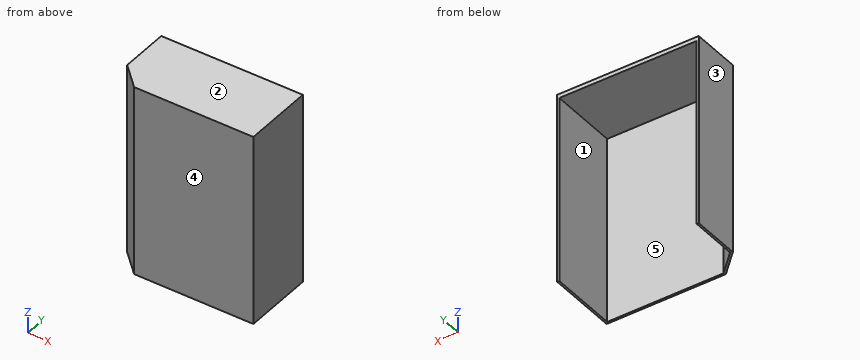
from build123d import *

# Parameters (mm, degrees)
F1_DEPTH = 900
F3_DEPTH = 20


with BuildPart() as f1:
    # F0 (on Top) → F1 (new body)
    with BuildSketch(Plane.XY):
        Polygon((0, 100), (0, 330), (-10, 330), (-10, 95.789346), (95.926052, -7.69314), (670, -7.69314), (670, 332.30686), (660, 332.30686), (660, 2.30686), (100, 2.30686), align=None)
    extrude(amount=F1_DEPTH)

    # F2 (on face) → F3 (join)
    with BuildSketch(Plane.XY.offset(900)):
        Polygon((670, 332.30686), (-10, 330), (-10, 95.789346), (95.926052, -7.69314), (670, -7.69314), align=None)
    extrude(amount=F3_DEPTH)


solid = f1.part
Here's how the part is built. I have some questions about the finished solid (model axes, mm). Face numbers are marked on the shaded views. A direction names the side the tool comes from. Give positions to 0.01 mm unless a question says otherwise; leave off trailing zeros. Order: outer loops, then holes, each group sorted by start corner. A loop starts at its lowest first (then second) coordinate and runs counter-clockwise, first axis right, second up. Notation, with made-up numbers: (-4.75, 6) -> (6.25, 6) arc R26 cw to (6.25, 26) -> close; hole circle Ø10 at (29.5, 12). An arc over 180 degrees is marked (long way). Use a Markdown table: item, result. Add a question column.
Item 1: Imagine slicing it at A-A on y = 229. Please give me the cut outline in (x, z), plus the area to 3 significant figures.
Item 2: Will these pins go through, and if not, where does the flat tip stop? pin 1 (3 mm diameter, centred on x = 111.5, y = 177.5, fed in from -Z); pin 2 (5 mm diameter, centred on x = 320.5, z = 785, fed in from +Y); pin 3 (5 mm diameter, centred on x = -5.5, z = 568.5, fed in from +Y).
Item 3: If we mould it in two halves opening along X, with no side actions, what happens to the marked faces 1, 2 and 3? For each: pulls with the +X half, pulls with the -X half, needs draft (parallel to the pull), parting line crosses it, or undercut.
Item 4: Imagine slicing it at B-B on z = 842. Please give me the cut outline in (x, y), plus the area to 3 significant figures.
Item 5: I need wall thicknesses on line 1 (X direction, y = 127, z = 623.5); line 2 (Y direction, x = 106, z = 616.5); line 3 (Z direction, x = 476.5, y = 151). Which ranges of each line are inside material? Lowest first, please.
Item 6: Imagine slicing it at D-D on x = 461. Please give me the cut outline in (y, z), plus the area to 3 significant figures.
Item 7: Imagine slicing it at C-C on x = 320.5. Please give me the cut outline in (y, z), plus the area to 3 significant figures.
Item 8: For the marked faces 4 and 5, which set-ups out of +Z, -Z, +X, -X, +Y, -Y let a thin tool reach every point of the face, with its end or its side?
Data:
| question | item | result |
|---|---|---|
| 1 | outline | (-10, 0) -> (0, 0) -> (0, 900) -> (660, 900) -> (660, 0) -> (670, 0) -> (670, 920) -> (-10, 920) -> close |
| 1 | area | 31,600 mm² |
| 2 | pin 1 | stops at z = 900 |
| 2 | pin 2 | stops at y = 2.31 |
| 2 | pin 3 | stops at y = 330 |
| 3 | face 1 | undercut |
| 3 | face 2 | needs draft |
| 3 | face 3 | pulls with the -X half |
| 4 | outline | (-10, 95.79) -> (95.93, -7.69) -> (670, -7.69) -> (670, 332.31) -> (660, 332.31) -> (660, 2.31) -> (100, 2.31) -> (0, 100) -> (0, 330) -> (-10, 330) -> close |
| 4 | area | 12,800 mm² |
| 5 | line 1 | x = -10 to 0, 660 to 670 |
| 5 | line 2 | y = -7.69 to 2.31 |
| 5 | line 3 | z = 900 to 920 |
| 6 | outline | (-7.69, 0) -> (2.31, 0) -> (2.31, 900) -> (331.6, 900) -> (331.6, 920) -> (-7.69, 920) -> close |
| 6 | area | 15,800 mm² |
| 7 | outline | (-7.69, 0) -> (2.31, 0) -> (2.31, 900) -> (331.12, 900) -> (331.12, 920) -> (-7.69, 920) -> close |
| 7 | area | 15,800 mm² |
| 8 | face 4 | +Z, -Z, +X, -X, -Y |
| 8 | face 5 | -Z, +Y |
